from build123d import *

# Parameters (mm, degrees)
SKETCH1_W           = 10.1
SKETCH1_H           = 25.6
BOSS_EXTRUDE1_DEPTH = 7.1
SKETCH2_W           = 0.5
SKETCH2_H           = 0.5
BOSS_EXTRUDE2_DEPTH = 4.2
SKETCH3_W           = 5
SKETCH3_H           = 2
CUT_EXTRUDE1_DEPTH  = 0.1


with BuildPart() as part:
    # Sketch1 → Boss-Extrude1 (new body)
    with BuildSketch(Plane(origin=(0, 0, 0), x_dir=(1, 0, 0), z_dir=(0, 1, 0))):
        Rectangle(SKETCH1_W, SKETCH1_H)
    extrude(amount=BOSS_EXTRUDE1_DEPTH)

    # Sketch2 → Boss-Extrude2 (add)
    with BuildSketch(Plane(origin=(0, 0, 0), x_dir=(1, 0, 0), z_dir=(0, 1, 0))):
        with Locations((3.85, -11.25)):
            Rectangle(SKETCH2_W, SKETCH2_H)
        with Locations((-3.85, -11.25)):
            Rectangle(SKETCH2_W, SKETCH2_H)
        with Locations((3.85, -8.75)):
            Rectangle(SKETCH2_W, SKETCH2_H)
        with Locations((3.85, -6.25)):
            Rectangle(SKETCH2_W, SKETCH2_H)
        with Locations((3.85, -3.75)):
            Rectangle(SKETCH2_W, SKETCH2_H)
        with Locations((3.85, -1.25)):
            Rectangle(SKETCH2_W, SKETCH2_H)
        with Locations((3.85, 1.25)):
            Rectangle(SKETCH2_W, SKETCH2_H)
        with Locations((3.85, 3.75)):
            Rectangle(SKETCH2_W, SKETCH2_H)
        with Locations((3.85, 6.25)):
            Rectangle(SKETCH2_W, SKETCH2_H)
        with Locations((3.85, 8.75)):
            Rectangle(SKETCH2_W, SKETCH2_H)
        with Locations((3.85, 11.25)):
            Rectangle(SKETCH2_W, SKETCH2_H)
        with Locations((-3.85, -8.75)):
            Rectangle(SKETCH2_W, SKETCH2_H)
        with Locations((-3.85, -6.25)):
            Rectangle(SKETCH2_W, SKETCH2_H)
        with Locations((-3.85, -3.75)):
            Rectangle(SKETCH2_W, SKETCH2_H)
        with Locations((-3.85, -1.25)):
            Rectangle(SKETCH2_W, SKETCH2_H)
        with Locations((-3.85, 1.25)):
            Rectangle(SKETCH2_W, SKETCH2_H)
        with Locations((-3.85, 3.75)):
            Rectangle(SKETCH2_W, SKETCH2_H)
        with Locations((-3.85, 6.25)):
            Rectangle(SKETCH2_W, SKETCH2_H)
        with Locations((-3.85, 8.75)):
            Rectangle(SKETCH2_W, SKETCH2_H)
        with Locations((-3.85, 11.25)):
            Rectangle(SKETCH2_W, SKETCH2_H)
    extrude(amount=-BOSS_EXTRUDE2_DEPTH)

    # Sketch3 → Cut-Extrude1 (cut)
    with BuildSketch(Plane(origin=(0, 7.1, 0), x_dir=(1, 0, 0), z_dir=(0, 1, 0))):
        with Locations((0, 9.1)):
            Rectangle(SKETCH3_W, SKETCH3_H)
        with Locations((0, 11.7)):
            Rectangle(SKETCH3_W, SKETCH3_H)
        with Locations((0, 6.5)):
            Rectangle(SKETCH3_W, SKETCH3_H)
        with Locations((0, 3.9)):
            Rectangle(SKETCH3_W, SKETCH3_H)
        with Locations((0, 1.3)):
            Rectangle(SKETCH3_W, SKETCH3_H)
        with Locations((0, -1.3)):
            Rectangle(SKETCH3_W, SKETCH3_H)
        with Locations((0, -3.9)):
            Rectangle(SKETCH3_W, SKETCH3_H)
        with Locations((0, -6.5)):
            Rectangle(SKETCH3_W, SKETCH3_H)
        with Locations((0, -9.1)):
            Rectangle(SKETCH3_W, SKETCH3_H)
        with Locations((0, -11.7)):
            Rectangle(SKETCH3_W, SKETCH3_H)
    extrude(amount=-CUT_EXTRUDE1_DEPTH, mode=Mode.SUBTRACT)


solid = part.part
Read the model definition and answer for the solid it produces. Units are mm, in the model's axes. A direction names the side the tool comes from. Round coordinates to 2 decimals unless told otherwise and drop trailing zeros. Order: outer loops, then holes, each group sorted by start corner. A loop starts at its lowest first (then second) coordinate and runs counter-clockwise, first axis right, second up. Notation, with made-up numbers: (78, 87.5) - (118, 87.5) arc R11 cw to (118, 97.5) - close; hole circle Ø9 at (16.5, -10). An arc over 180 degrees is marked (long way). Use one line per item in the form item = value. Start each with the question number.
(1) The part is cut by section C-C (z = 11.25). Give the vertices of the cut face in (x, y), then the cut area to 3 significant figures.
(2) The part is cut by section A-A (z = -7). Give the vertices of the cut face in (x, y), then the cut area to 3 significant figures.
(3) The part is cut by section B-B (y = -0.75). Count the separate pieces of the cut face and the enclosed holes in it, then the cut area to 3 significant figures.
(4) Flat-ended cylindrical pins translate along their axes: pin 1 Ø0.5 at (x, y) = (-4, -2.5) entering from -Z; pin 2 Ø0.6 at (y, z) = (-2, -4) entering from -X. Find the tip coordinate at first contact, or state that the pin passes through.
(5) Find the intervals of material crossed by line 1 along X through (y, z) = (-3.5, -6.25); line 2 along Y through (x, z) = (1, 9.75); line 3 along Y through (x, z) = (-3.25, 1.5), in increasing order. Write a range as from..to.
(6) For faces 1 (the face through (0, 7, -7)), 2 (the face through (-5.05, 4, 0)), determine the directions among +Z, -Z, +X, -X, +Y, -Y from which every point of the face is accessible in a straight line to the end or side of a thin tool.
(7) Determine the mould class of faces 3 (the face through (0, 7, -9)), 4 (the face through (0, 4, -12.8)), 5 (the face through (5.05, 4, 0)), 6 (the face through (0, 4, 12.8)) for opening direction Z: +Z half, -Z half, draft (parallel to the pull), parting line (faces both ways), or undercut.
Checked values:
q1.outline = (-5.05, 0) - (-4.1, 0) - (-4.1, -4.2) - (-3.6, -4.2) - (-3.6, 0) - (3.6, 0) - (3.6, -4.2) - (4.1, -4.2) - (4.1, 0) - (5.05, 0) - (5.05, 7.1) - (2.5, 7.1) - (2.5, 7) - (-2.5, 7) - (-2.5, 7.1) - (-5.05, 7.1) - close
q1.area = 75.4 mm^2
q2.outline = (-5.05, 0) - (5.05, 0) - (5.05, 7.1) - (2.5, 7.1) - (2.5, 7) - (-2.5, 7) - (-2.5, 7.1) - (-5.05, 7.1) - close
q2.area = 71.2 mm^2
q3.separate_pieces = 20
q3.enclosed_holes = 0
q3.area = 5.00 mm^2
q4.pin_1 = -11.5
q4.pin_2 = -4.1
q5.line_1 = -4.1..-3.6, 3.6..4.1
q5.line_2 = 0..7
q5.line_3 = 0..7.1
q6.face_1 = +Y
q6.face_2 = +Z, -Z, -X, +Y, -Y
q7.face_3 = undercut
q7.face_4 = -Z half
q7.face_5 = draft
q7.face_6 = +Z half
